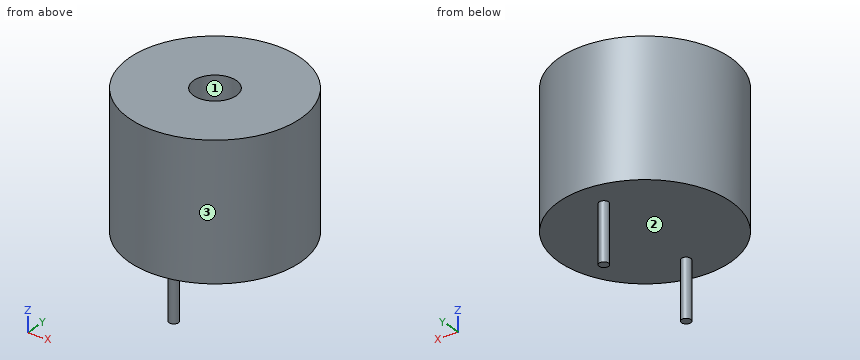
from build123d import *

# Parameters (mm, degrees)
F0_R     = 6
F1_DEPTH = 4.7
F2_R     = 1.5
F3_DEPTH = 2
F4_R     = 0.33
F5_DEPTH = 4


with BuildPart() as f1:
    # F0 (on Top) → F1 (new body, symmetric)
    with BuildSketch(Plane.XY):
        Circle(F0_R)
    extrude(amount=F1_DEPTH, both=True)

    # F2 (on face) → F3 (cut)
    with BuildSketch(Plane.XY.offset(4.7)):
        Circle(F2_R)
    extrude(amount=-F3_DEPTH, mode=Mode.SUBTRACT)

    # F4 (on face) → F5 (join)
    with BuildSketch(Plane(origin=(0, 0, -4.7), x_dir=(1, 0, 0), z_dir=(0, 0, -1))):
        with Locations((0, 4)):
            Circle(F4_R)
        with Locations((0, -4)):
            Circle(F4_R)
    extrude(amount=F5_DEPTH)


solid = f1.part
The model under review builds one solid part; all positions refer to its coordinate system, in mm. Face numbers are marked on the shaded views. Coordinates: 2 decimals unless noted, no trailing zeros. Loops run counter-clockwise (first coordinate to the right, second up) from the corner with the lowest first, then second, coordinate; pieces in that order, holes last. Notation, with made-up numbers: (12.5, -23.5) -> (52.5, -23.5) arc R19 ccw to (52.5, 13.5) -> close; hole circle Ø11 at (44, -21.75). An arc over 180 degrees is marked (long way). Use a Markdown table: item, result. Add a question column.
1. Add section C-C on z = -3. Write out the cut boundary in (x, y), plus the area to 3 significant figures.
2. Add section D-D on y = -4. Write out the cut boundary in (x, z), plus the area to 3 significant figures.
3. Draft analysis for pull direction X (two halves, no side actions). For the marked faces 1, 2 and 3, state which applies: pulls with the +X half, pulls with the -X half, needs draft (parallel to the pull), parting line crosses it, or undercut.
4. Clearance check with flat-ended pins moving along their axes: pin 1 Ø4 at (x, y) = (0, 0) entering from -Z; pin 2 Ø1 at (y, z) = (4.5, -3) entering from +X; pin 3 Ø1.5 at (x, z) = (-3.5, 1.5) entering from -Y; pin 4 Ø1.5 at (x, z) = (-3.5, -6) entering from +Y. State where each tip first meets the part, or that it passes through.
5. To check wall thickness, follow line 1 (Y direction, x = 0, z = 3.4); line 2 (Z direction, x = -1.5, y = -5); line 3 (Z direction, x = -0.25, y = -0.25). State the ranges of each line that lie inside material, in increasing order.
6. Add section A-A on x = 0. Write out the cut boundary in (y, z), plus the area to 3 significant figures.
7. Add section B-B on y = 0. Write out the cut boundary in (x, z).
Returned:
| question | item | result |
|---|---|---|
| 1 | outline | circle Ø12 at (0, 0) |
| 1 | area | 113 mm² |
| 2 | outline | (-4.47, -4.7) -> (-0.33, -4.7) -> (-0.33, -8.7) -> (0.33, -8.7) -> (0.33, -4.7) -> (4.47, -4.7) -> (4.47, 4.7) -> (-4.47, 4.7) -> close |
| 2 | area | 86.7 mm² |
| 3 | face 1 | undercut |
| 3 | face 2 | needs draft |
| 3 | face 3 | parting line crosses it |
| 4 | pin 1 | stops at z = -4.7 |
| 4 | pin 2 | stops at x = 4.47 |
| 4 | pin 3 | stops at y = -5.33 |
| 4 | pin 4 | passes through |
| 5 | line 1 | y = -6 to -1.5, 1.5 to 6 |
| 5 | line 2 | z = -4.7 to 4.7 |
| 5 | line 3 | z = -4.7 to 2.7 |
| 6 | outline | (-6, -4.7) -> (-4.33, -4.7) -> (-4.33, -8.7) -> (-3.67, -8.7) -> (-3.67, -4.7) -> (3.67, -4.7) -> (3.67, -8.7) -> (4.33, -8.7) -> (4.33, -4.7) -> (6, -4.7) -> (6, 4.7) -> (1.5, 4.7) -> (1.5, 2.7) -> (-1.5, 2.7) -> (-1.5, 4.7) -> (-6, 4.7) -> close |
| 6 | area | 112 mm² |
| 7 | outline | (-6, -4.7) -> (6, -4.7) -> (6, 4.7) -> (1.5, 4.7) -> (1.5, 2.7) -> (-1.5, 2.7) -> (-1.5, 4.7) -> (-6, 4.7) -> close |
